from build123d import *

# Parameters (mm, degrees)
EXTRUDE_1_DEPTH      = 15
SKETCH_2_R           = 5
CUT_EXTRUDE_1_DEPTH  = 44.011626335
SKETCH_3_R           = 4.781082329
EXTRUDE_2_DEPTH      = 10
MIRROR_START         = 29
MIRROR_1_OUTLINE_W   = 35
MIRROR_1_OUTLINE_H   = 30
MIRROR_1_DEPTH       = 15
MIRROR_START_2       = 20
MIRROR_1_2_OUTLINE_W = 5
MIRROR_1_2_OUTLINE_H = 30
MIRROR_1_2_DEPTH     = 9
MIRROR_START_3       = 44
MIRROR_1_3_OUTLINE_R = 4.781082329
MIRROR_1_3_DEPTH     = 10


# Read off the part's stored shape, not the designer's step: the mirror step
with BuildPart() as part:
    # Sketch 1 → Extrude 1 (new, symmetric)
    with BuildSketch(Plane.XY):
        Polygon((-17.5, -20), (17.5, -20), (17.5, 20), (12.5, 20), (12.5, -5), (-12.5, -5), (-12.5, 20), (-17.5, 20), align=None)
    extrude(amount=EXTRUDE_1_DEPTH, both=True)

    # Sketch 2 → Cut-Extrude 1 (cut, through all)
    with BuildSketch(Plane(origin=(17.5, 0, 0), x_dir=(0, 0, -1), z_dir=(1, 0, 0))):
        with Locations((0, 12)):
            Circle(SKETCH_2_R)
    extrude(amount=-CUT_EXTRUDE_1_DEPTH, mode=Mode.SUBTRACT)

    # Sketch 3 → Extrude 2 (add)
    with BuildSketch(Plane.XZ.offset(20)):
        with Locations(Location((0, 0, 0), (0, 0, 90))):
            Circle(SKETCH_3_R)
    extrude(amount=EXTRUDE_2_DEPTH)



with BuildPart() as body_2:
    # Mirror 1 outline → Mirror 1 (new body)
    with BuildSketch(Plane(origin=(0, 0, 0), x_dir=(1, 0, 0), z_dir=(0, 1, 0)).offset(MIRROR_START)):
        Rectangle(MIRROR_1_OUTLINE_W, MIRROR_1_OUTLINE_H)
    extrude(amount=MIRROR_1_DEPTH)


with BuildPart() as part_1:
    add(part.part)

    add(body_2.part)  # Mirror 1 2 merges body 2
    # Mirror 1 2 outline → Mirror 1 2 (add)
    with BuildSketch(Plane(origin=(0, 0, 0), x_dir=(1, 0, 0), z_dir=(0, 1, 0)).offset(MIRROR_START_2)):
        with Locations((15, 0)):
            Rectangle(MIRROR_1_2_OUTLINE_W, MIRROR_1_2_OUTLINE_H)
        with Locations((-15, 0)):
            Rectangle(MIRROR_1_2_OUTLINE_W, MIRROR_1_2_OUTLINE_H)
    extrude(amount=MIRROR_1_2_DEPTH)

    # Mirror 1 3 outline → Mirror 1 3 (add)
    with BuildSketch(Plane(origin=(0, 0, 0), x_dir=(1, 0, 0), z_dir=(0, 1, 0)).offset(MIRROR_START_3)):
        Circle(MIRROR_1_3_OUTLINE_R)
    extrude(amount=MIRROR_1_3_DEPTH)


solid = part_1.part
Read the model definition and answer for the solid it produces. Units are mm, in the model's axes. A direction names the side the tool comes from. Coordinates: 2 decimals unless noted, no trailing zeros. Loops run counter-clockwise (first coordinate to the right, second up) from the corner with the lowest first, then second, coordinate; pieces in that order, holes last.
Q1. The part is cut by section B-B on z = 8.5. Write down the section's boundary in (x, y), and give its area (3 significant figures).
Q2. The mould has two halves that part along X. Classify faces 1 (the face through (-17.5, 12, 7)), 2 (the face through (12.5, 8, 4)), 3 (the face through (-16, 12, 15)), 4 (the face through (-12.5, 8, 4)): +X half, -X half, draft (parallel to the pull), parting line (faces both ways), or undercut.
Q3. The part is cut by section D-D on z = 0. Write down the section's boundary in (x, y), and give its area (3 significant figures).
Q4. The part is cut by section C-C on y = 12. Write down the section's boundary in (x, z), and give its area (3 significant figures).
Q5. The part is cut by section A-A on x = 0. Write down the section's boundary in (y, z).
Q6. Each of these flat-tipped pins is pushed along its axis until it touches: pin 1 Ø1 at (x, z) = (13.5, -5.5) entering from -Y; pin 2 Ø3 at (x, z) = (7.5, -0.5) entering from +Y. Where does it stop, or does it pass through?
Q7. Consider probe 1 along X at (y, z) = (11, 13); probe 2 along Y at (x, z) = (15.15, 0); probe 3 along Y at (x, z) = (-7, 4). Determine where each line is inside the solid, lowest interval first.
Q8. Which of the six approach directions +Z, -Z, +X, -X, +Y, -Y give full straight-line access (tool end or side, diameter ignored) to faces 5 (the face through (0, -30, 0)), 6 (the face through (-0.62, 48.93, -4.74)), 7 (the face through (4, -20, 4)), 8 (the face through (0, 29, 0))?
Results below:
1. outline: (-17.5, -20) - (17.5, -20) - (17.5, 44) - (-17.5, 44) - close; hole (-12.5, -5) - (12.5, -5) - (12.5, 29) - (-12.5, 29) - close
1. area: 1,390 mm2
2. face 1: -X half
2. face 2: undercut
2. face 3: draft
2. face 4: undercut
3. outline: (-17.5, -20) - (-4.78, -20) - (-4.78, -30) - (4.78, -30) - (4.78, -20) - (17.5, -20) - (17.5, 7) - (12.5, 7) - (12.5, -5) - (-12.5, -5) - (-12.5, 7) - (-17.5, 7) - close; (-17.5, 17) - (-12.5, 17) - (-12.5, 29) - (12.5, 29) - (12.5, 17) - (17.5, 17) - (17.5, 44) - (4.78, 44) - (4.78, 54) - (-4.78, 54) - (-4.78, 44) - (-17.5, 44) - close
3. area: 1,480 mm2
4. outline: (-17.5, -15) - (-12.5, -15) - (-12.5, -5) - (-17.5, -5) - close; (-17.5, 5) - (-12.5, 5) - (-12.5, 15) - (-17.5, 15) - close; (12.5, -15) - (17.5, -15) - (17.5, -5) - (12.5, -5) - close; (12.5, 5) - (17.5, 5) - (17.5, 15) - (12.5, 15) - close
4. area: 200 mm2
5. outline: (-30, -4.78) - (-20, -4.78) - (-20, -15) - (-5, -15) - (-5, 15) - (-20, 15) - (-20, 4.78) - (-30, 4.78) - close; (29, -15) - (44, -15) - (44, -4.78) - (54, -4.78) - (54, 4.78) - (44, 4.78) - (44, 15) - (29, 15) - close
6. pin 1: stops at y = -20
6. pin 2: stops at y = 44
7. probe 1: x = -17.5 to -12.5, 12.5 to 17.5
7. probe 2: y = -20 to 7, 17 to 44
7. probe 3: y = -20 to -5, 29 to 44
8. face 5: +Z, -Z, +X, -X, -Y
8. face 6: +Y
8. face 7: -Y
8. face 8: +Z, -Z
